Check sheet for the modelled part. Datum: model origin and axes. Units: mm. A direction names the side the tool comes from. Coordinates: 2 decimals unless noted, no trailing zeros. Order: outer loops, then holes, each group sorted by start corner. A loop starts at its lowest first (then second) coordinate and runs counter-clockwise, first axis right, second up. Notation, with made-up numbers: M -18.75,-6.75 L 32.25,-6.75 A17 ccw 32.25,9.25 Z; hole C 73,24 d1. An arc over 180 degrees is marked long. Answer in a Markdown table with one row per item. Add a question column.
Autodesk Inventor part; units mm, degrees
ref_plane "YZ Plane" through (0, 0, 0) normal (1, 0, 0) x (0, 1, 0)
ref_plane "XZ Plane" through (0, 0, 0) normal (0, 1, 0) x (-1, 0, 0)
ref_plane "XY Plane" through (0, 0, 0) normal (0, 0, 1) x (1, 0, 0)
sketch "Эскиз1" plane through (0, 0, 0) normal (0, 0, 1) x (1, 0, 0)
  arc A0 (0, -25) -> (0, 25) centre (0, 0) ccw
  arc A1 (0, -20) -> (0, 20) centre (0, 0) ccw
  line L0 (0, 25) -> (0, 20)
  line L1 (0, -20) -> (0, -25)
  line L2 (0, -35) -> (0, 35)
  dimension "d0" = 20
  dimension "d1" = 25
revolve "Вращение1" add sketch "Эскиз1" angle 360 about axis through (0, -10, 0) along (0, 1, 0) contours L1 A1 L0 A0
sketch "Эскиз2" plane through (0, 0, 0) normal (0, 0, 1) x (1, 0, 0)
  circle A0 centre (0, 0) radius 13
  dimension "d3" = 26
extrude "Выдавливание1" cut sketch "Эскиз2" against normal through all
sketch "Эскиз3" plane through (0, 0, 0) normal (0, 1, 0) x (-1, 0, 0)
  arc A0 (13, -21.3542) -> (-13, -21.3542) centre (0, 0) ccw
  line L0 (13, 10) -> (-13, 10)
  line L1 (-13, 10) -> (-13, 25)
  line L2 (-13, 25) -> (13, 25)
  line L3 (13, 25) -> (13, 10)
  dimension "d6" = 10
  dimension "d7" = 26
  dimension "d9" = 13
extrude "Выдавливание2" cut sketch "Эскиз3" along normal through all both and the other way through all
1. Section check B-B on x = 0. Enter the section's corners in (y, z).
2. Section check C-C on z = 17. Enter the section's corners in (x, y), then the cut area to 3 significant figures.
3. Scan lines: line 1 (X direction, y = 1.5, z = 14); line 2 (X direction, y = 0, z = -19.5); line 3 (Y direction, x = -8, z = 5.5). Record each from-to range of solid material in increasing order.
4. Release check for a two-part mould opening along X. For faces 3 (the flat face through (0, 18, 10)), 4 (the flat face through (-13, 0, 16)) record: released by +X, released by -X, zero draft, split by the parting line, or undercut.
5. Set-up check for faces 1 (the flat face through (13, 0, 16)), 2 (the cylindrical face through (-10.316, -7.91, -18.233)): record each of +Z, -Z, +X, -X, +Y, -Y from which the full face is reachable in a straight line by a thin tool's end or side.
6. Go/stop test with flat-tipped pins: pin 1 Ø3 at (x, z) = (-1.5, -19) entering from -Y; pin 2 Ø1 at (y, z) = (-18, -8.5) entering from -X; pin 3 Ø8 at (x, z) = (11, -9) entering from +Y. Record where each tip stops, or that it passes through.
7. Section check D-D on y = 17. Enter the section's corners in (x, z).
8. Section check A-A on y = -3.5. Enter the section's corners in (x, z), then the cut area to 3 significant figures.
Result sheet:
| question | item | result |
|---|---|---|
| 1 | outline | M -22.91,10 A25 ccw -13,-21.35 L -13,-15.2 A20 cw -17.32,10 Z; M 13,-21.35 A25 ccw 22.91,10 L 17.32,10 A20 cw 13,-15.2 Z |
| 2 | outline | M -13,-12.92 L -13,12.92 A18.33 ccw Z; M 13,-12.92 A18.33 ccw 13,12.92 Z |
| 2 | area | 190 mm^2 |
| 3 | line 1 | -20.66 to -14.2, 14.2 to 20.66 |
| 3 | line 2 | -15.64 to -13, 13 to 15.64 |
| 3 | line 3 | -23.04 to -17.49, 17.49 to 23.04 |
| 4 | face 3 | undercut |
| 4 | face 4 | undercut |
| 5 | face 1 | +Z, +Y, -Y |
| 5 | face 2 | +Z, -Z |
| 6 | pin 1 | y = -17.8 |
| 6 | pin 2 | x = -15.76 |
| 6 | pin 3 | y = 22.82 |
| 7 | outline | M -13,10 L -13,12.92 A18.33 ccw long 13,12.92 L 13,10 L 3.32,10 A10.54 cw long -3.32,10 Z |
| 8 | outline | M -13,14.79 L -13,21.07 A24.75 ccw -12.52,-21.35 L -12.52,-15.2 A19.69 cw Z; M 12.52,-21.35 A24.75 ccw 13,21.07 L 13,14.79 A19.69 cw 12.52,-15.2 Z |
| 8 | area | 431 mm^2 |
